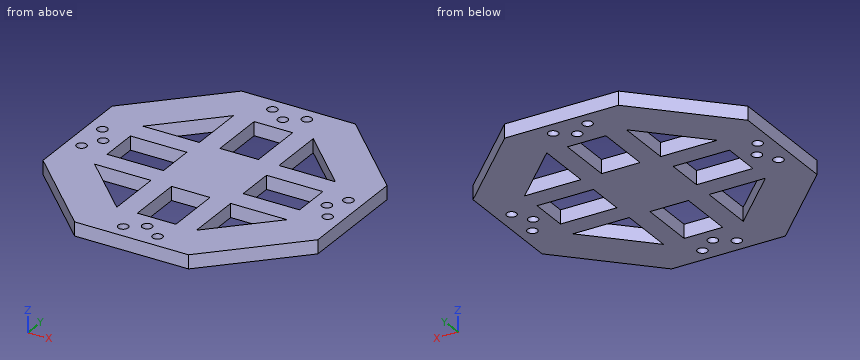
```python
from build123d import *

# Parameters (mm, degrees)
F1_DEPTH  = 5.08
F3_DEPTH  = 5.081
F4_W      = 7.62
F4_H      = 20.830565722
F4_H_2    = 7.62
F4_W_2    = 20.830565722
F4_W_3    = 14.218868556
F4_H_3    = 14.218868556
F5_DEPTH  = 5.08
F6_R      = 1.8415
F10_DEPTH = 5.081
F7_R      = 1.8415
F11_DEPTH = 5.081
F8_R      = 1.8415
F12_DEPTH = 5.081
F9_R      = 1.8415
F13_DEPTH = 5.081
F14_W     = 14.218868556
F14_H     = 14.218868556
F15_DEPTH = 5.08


with BuildPart() as f1:
    # F0 (on Top) → F1 (new body)
    with BuildSketch(Plane.XY):
        Polygon((21.0420489686, 50.8), (-21.0420489686, 50.8), (-50.8, 21.0420489686), (-50.8, -21.0420489686), (-21.0420489686, -50.8), (21.0420489686, -50.8), (50.8, -21.0420489686), (50.8, 21.0420489686), align=None)
    extrude(amount=F1_DEPTH)

    # F2 (on face) → F3 (cut, through all)
    with BuildSketch(Plane.XY.offset(5.08)):
        Polygon((14.729434278, 35.56), (-14.729434278, 35.56), (-35.56, 14.729434278), (-35.56, -14.729434278), (-14.729434278, -35.56), (14.729434278, -35.56), (35.56, -14.729434278), (35.56, 14.729434278), align=None)
    extrude(amount=-F3_DEPTH, mode=Mode.SUBTRACT)

    # F4 (on face) → F5 (join)
    with BuildSketch(Plane.XY.offset(5.08)):
        with Locations((-10.919434278, 25.144717139)):
            Rectangle(F4_W, F4_H)
        with Locations((-10.919434278, 10.919434278)):
            Rectangle(F4_W, F4_H_2)
        with Locations((-25.144717139, 10.919434278)):
            Rectangle(F4_W_2, F4_H_2)
        with Locations((0, 10.919434278)):
            Rectangle(F4_W_3, F4_H_2)
        with Locations((-10.919434278, 0)):
            Rectangle(F4_W, F4_H_3)
        with Locations((10.919434278, 10.919434278)):
            Rectangle(F4_W, F4_H_2)
        with Locations((10.919434278, 25.144717139)):
            Rectangle(F4_W, F4_H)
        with Locations((-10.919434278, -10.919434278)):
            Rectangle(F4_W, F4_H_2)
        with Locations((-25.144717139, -10.919434278)):
            Rectangle(F4_W_2, F4_H_2)
        with Locations((0, -10.919434278)):
            Rectangle(F4_W_3, F4_H_2)
        with Locations((10.919434278, 0)):
            Rectangle(F4_W, F4_H_3)
        with Locations((25.144717139, 10.919434278)):
            Rectangle(F4_W_2, F4_H_2)
        with Locations((-10.919434278, -25.144717139)):
            Rectangle(F4_W, F4_H)
        with Locations((10.919434278, -10.919434278)):
            Rectangle(F4_W, F4_H_2)
        with Locations((10.919434278, -25.144717139)):
            Rectangle(F4_W, F4_H)
        with Locations((25.144717139, -10.919434278)):
            Rectangle(F4_W_2, F4_H_2)
    extrude(amount=-F5_DEPTH)

    # F6 (on face) → F10 (cut, through all)
    with BuildSketch(Plane.XY.offset(5.08)):
        with Locations((45.466, 6.35)):
            Circle(F6_R)
        with Locations((45.466, -6.35)):
            Circle(F6_R)
        with Locations((41.3512, 0)):
            Circle(F6_R)
    extrude(amount=-F10_DEPTH, mode=Mode.SUBTRACT)

    # F7 (on face) → F11 (cut, through all)
    with BuildSketch(Plane.XY.offset(5.08)):
        with Locations((-6.3550683909, 45.466)):
            Circle(F7_R)
        with Locations((6.3449316091, 45.466)):
            Circle(F7_R)
        with Locations((-0.0050683909, 41.3512)):
            Circle(F7_R)
    extrude(amount=-F11_DEPTH, mode=Mode.SUBTRACT)

    # F8 (on face) → F12 (cut, through all)
    with BuildSketch(Plane.XY.offset(5.08)):
        with Locations((-45.466, -6.3510387499)):
            Circle(F8_R)
        with Locations((-45.466, 6.3489612501)):
            Circle(F8_R)
        with Locations((-41.3512, -0.0010387499)):
            Circle(F8_R)
    extrude(amount=-F12_DEPTH, mode=Mode.SUBTRACT)

    # F9 (on face) → F13 (cut, through all)
    with BuildSketch(Plane.XY.offset(5.08)):
        with Locations((6.3503286729, -45.466)):
            Circle(F9_R)
        with Locations((-6.3496713271, -45.466)):
            Circle(F9_R)
        with Locations((0.0003286729, -41.3512)):
            Circle(F9_R)
    extrude(amount=-F13_DEPTH, mode=Mode.SUBTRACT)

    # F14 (on face) → F15 (join)
    with BuildSketch(Plane.XY.offset(5.08)):
        Rectangle(F14_W, F14_H)
    extrude(amount=-F15_DEPTH)


solid = f1.part
```
Model file for the job. Use its own axes, mm. Coordinates: 2 decimals unless noted, no trailing zeros. Order: outer loops, then holes, each group sorted by start corner. A loop starts at its lowest first (then second) coordinate and runs counter-clockwise, first axis right, second up. Notation, with made-up numbers: (71, 19.5) - (124, 19.5) arc R26 cw to (124, 41.5) - close; hole circle Ø11 at (10, 30.25). An arc over 180 degrees is marked (long way). Return JSON: item names as keys, results as strings. Group by question number.
1) Saw through at B-B, the plane x = 17.5. Write the cut outline in (y, z).
2) Saw through at A-A, the plane y = -29. Write the cut outline in (x, z), plus the area to 3 significant figures.
3) Flat gauge pins, fed straight in: P1, Ø4, axis at x = 12.5, y = -0.5, coming from the -Z side; P2, Ø4, axis at x = 32, y = 4.5, coming from the -Z side; P3, Ø1.5, axis at y = -25, z = 1.5, coming from the -X side; P4, Ø1.5, axis at x = -22.5, z = 3, coming from the -Y side. Where does each tip first touch, or does it go through?
4) Probe line 1 (X direction, y = -8, z = 1.7); line 2 (Y direction, x = -23.5, z = 0.6); line 3 (X direction, y = 25, z = 0.2). List the from-to ranges inside material, lowest first. Write a range as from..to.
5) Saw through at C-C, the plane z = 2.05. Count the separate pieces of the cut face and the enclosed holes in it, plus the area to 3 significant figures.
Values found:
{
 "1": {"outline": "(-50.8, 0) - (-32.79, 0) - (-32.79, 5.08) - (-50.8, 5.08) - close; (-14.73, 0) - (-7.11, 0) - (-7.11, 5.08) - (-14.73, 5.08) - close; (7.11, 0) - (14.73, 0) - (14.73, 5.08) - (7.11, 5.08) - close; (32.79, 0) - (50.8, 0) - (50.8, 5.08) - (32.79, 5.08) - close"},
 "2": {"outline": "(-42.84, 0) - (-21.29, 0) - (-21.29, 5.08) - (-42.84, 5.08) - close; (-14.73, 0) - (-7.11, 0) - (-7.11, 5.08) - (-14.73, 5.08) - close; (7.11, 0) - (14.73, 0) - (14.73, 5.08) - (7.11, 5.08) - close; (21.29, 0) - (42.84, 0) - (42.84, 5.08) - (21.29, 5.08) - close", "area": "296 mm²"},
 "3": {"P1": "stops at z = 0", "P2": "passes through", "P3": "stops at x = -47.59", "P4": "stops at y = -50.09"},
 "4": {"line 1": "x = -50.8..-46.29, -44.65..44.65, 46.28..50.8", "line 2": "y = -48.34..-26.79, -14.73..-7.11, 7.11..14.73, 26.79..48.34", "line 3": "x = -46.84..-25.29, -14.73..-7.11, 7.11..14.73, 25.29..46.84"},
 "5": {"separate pieces": "1", "enclosed holes": "20", "area": "6,370 mm²"}
}
